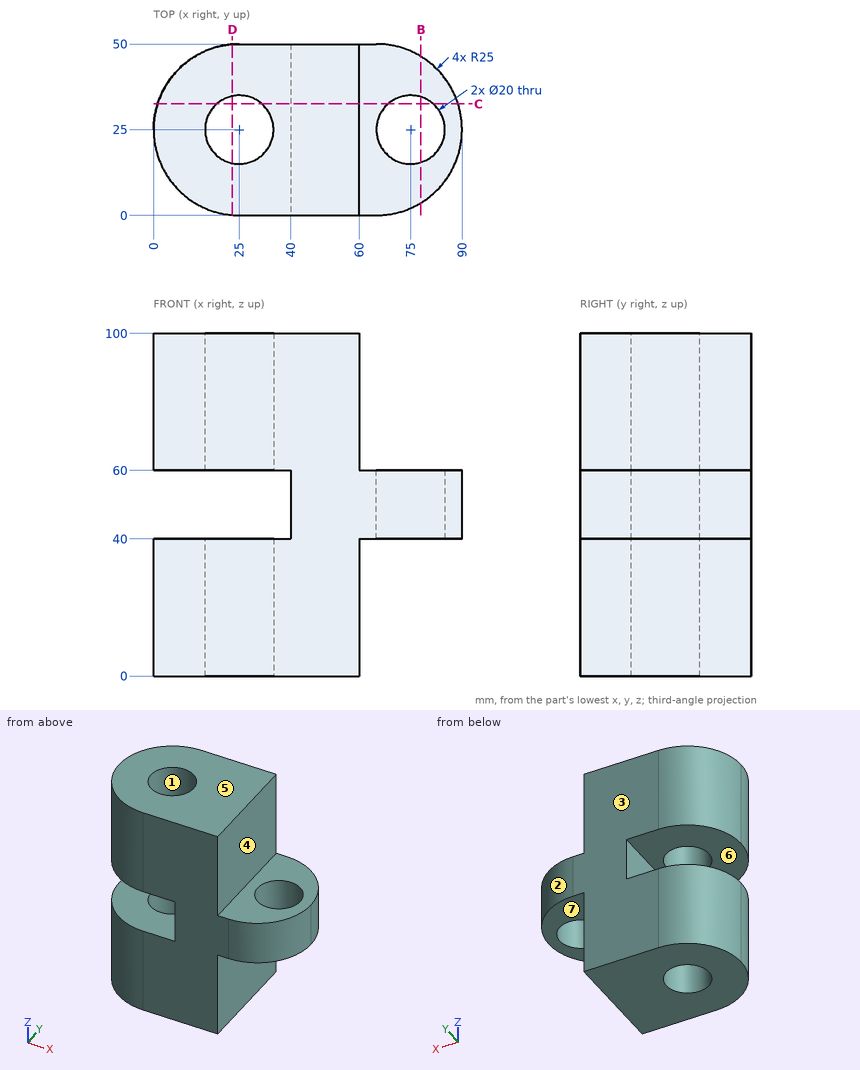
Could you check a few things on this drawing? It's one solid part, dimensions in mm from its lowest x, y, z. A direction names the side the tool comes from. Round coordinates to 2 decimals unless told otherwise and drop trailing zeros. Write each loop counter-clockwise with the first axis right and the second up, starting at its lowest first coordinate (ties: lowest second). Pieces come first, ordered by that corner, then holes.
Q1. Please list where these lines run through material, in increasing order: probe 1 along Z at (x, y) = (13.5, 20); probe 2 along Y at (x, z) = (25, 17); probe 3 along Z at (x, y) = (64, 37.5).
Q2. If we section it at D-D on x = 23: Write out the boundary of the cut face in (y, z).
Q3. If we section it at C-C on y = 32.5: Write out the boundary of the cut face in (x, z), plus the area to 3 significant figures.
Q4. If we mould it in two halves opening along X, with no side actions, what happens to the marked faces 1, 2 and 3? For each: +X half, -X half, draft (parallel to the pull), parting line (faces both ways), or undercut.
Q5. Will these pins go through, and if not, where does the flat tip stop? P1, Ø5, axis at y = 7, z = 68.5, coming from the +X side; P2, Ø5, axis at x = 70, y = 13.5, coming from the +Z side; P3, Ø24, axis at x = 80.5, y = 14, coming from the -Z side.
Q6. If we section it at B-B on x = 78: Write out the boundary of the cut face in (y, z), plus the area to 3 significant figures.
Q7. Which directions (+Z, -Z, +X, -X, +Y, -Y) give clear straight access to the entire face, cutting with the end or side of a thin tool? Please do the marked faces 4, 5, 6 and 7.
Answer below:
1. probe 1: z = 0 to 40, 60 to 100
1. probe 2: y = 0 to 15, 35 to 50
1. probe 3: z = 40 to 60
2. outline: (0.08, 0) - (15.2, 0) - (15.2, 40) - (0.08, 40) - close; (0.08, 60) - (15.2, 60) - (15.2, 100) - (0.08, 100) - close; (34.8, 0) - (49.92, 0) - (49.92, 40) - (34.8, 40) - close; (34.8, 60) - (49.92, 60) - (49.92, 100) - (34.8, 100) - close
3. outline: (1.15, 0) - (18.39, 0) - (18.39, 40) - (1.15, 40) - close; (1.15, 60) - (18.39, 60) - (18.39, 100) - (1.15, 100) - close; (31.61, 0) - (60, 0) - (60, 40) - (68.39, 40) - (68.39, 60) - (60, 60) - (60, 100) - (31.61, 100) - (31.61, 60) - (40, 60) - (40, 40) - (31.61, 40) - close; (81.61, 40) - (88.85, 40) - (88.85, 60) - (81.61, 60) - close
3. area: 4,360 mm2
4. face 1: undercut
4. face 2: +X half
4. face 3: draft
5. P1: stops at x = 60
5. P2: stops at z = 60
5. P3: stops at z = 40
6. outline: (3.65, 40) - (15.46, 40) - (15.46, 60) - (3.65, 60) - close; (34.54, 40) - (46.35, 40) - (46.35, 60) - (34.54, 60) - close
6. area: 473 mm2
7. face 4: +Z, +X, +Y, -Y
7. face 5: +Z, +X, -X, +Y, -Y
7. face 6: -X, +Y, -Y
7. face 7: -Z, +X, +Y, -Y
